Design review of the part built by this model. Coordinates are the model's own, in mm. Give positions to 0.01 mm unless a question says otherwise; leave off trailing zeros. Order: outer loops, then holes, each group sorted by start corner. A loop starts at its lowest first (then second) coordinate and runs counter-clockwise, first axis right, second up. Notation, with made-up numbers: (63.25, -35.5) -> (117.25, -35.5) arc R16 ccw to (117.25, -8.5) -> close; hole circle Ø7 at (-33, 64). An arc over 180 degrees is marked (long way). One line per item, written item: value.
from build123d import *

# Parameters (mm, degrees)
SKETCH1_R          = 16.891
EXTRUDE1_DEPTH     = 7.62
SKETCH2_R          = 8.636
CUT_EXTRUDE4_DEPTH = 26.073415443
SKETCH3_R          = 2.1844
CUT_EXTRUDE6_DEPTH = 7.62
CIRPATTERN1_COUNT  = 6


with BuildPart() as part:
    # Sketch1 → Extrude1 (new body)
    with BuildSketch(Plane(origin=(0, 0, 0), x_dir=(1, 0, 0), z_dir=(0, 1, 0))):
        with Locations(Location((0, 0, 0), (0, 0, 90))):
            Circle(SKETCH1_R)
    extrude(amount=EXTRUDE1_DEPTH)

    # Sketch2 → Cut-Extrude4 (cut, through all)
    with BuildSketch(Plane(origin=(0, 0, 0), x_dir=(1, 0, 0), z_dir=(0, 1, 0))):
        with Locations(Location((0, 0, 0), (0, 0, 90))):
            Circle(SKETCH2_R)
    extrude(amount=CUT_EXTRUDE4_DEPTH, mode=Mode.SUBTRACT)

    # Sketch3 → Cut-Extrude6 (cut)
    with BuildSketch(Plane(origin=(0, 0, 0), x_dir=(1, 0, 0), z_dir=(0, 1, 0))):
        with Locations(Location((0, 13.462, 0), (0, 0, 90))):
            Circle(SKETCH3_R)
    cut_extrude6 = extrude(amount=CUT_EXTRUDE6_DEPTH, mode=Mode.SUBTRACT)

    # CirPattern1: Cut-Extrude6 ×6 about axis
    cirpattern1_axis = Axis((0, 0, 0), (0, 1, 0))
    for i in range(1, CIRPATTERN1_COUNT):
        add(cut_extrude6.rotate(cirpattern1_axis, i * 360 / CIRPATTERN1_COUNT), mode=Mode.SUBTRACT)


solid = part.part
Item 1: Add section C-C on z = 0. Give the boundary of the cut face in (x, y), plus the area to 3 significant figures.
Returned:
outline: (-16.89, 0) -> (-8.64, 0) -> (-8.64, 7.62) -> (-16.89, 7.62) -> close; (8.64, 0) -> (16.89, 0) -> (16.89, 7.62) -> (8.64, 7.62) -> close
area: 126 mm²
Item 2: Add section D-D on x = -5.5. Give the boundary of the cut face in (y, z), plus the area to 3 significant figures.
Returned:
outline: (0, -15.97) -> (7.62, -15.97) -> (7.62, -6.66) -> (0, -6.66) -> close; (0, 6.66) -> (7.62, 6.66) -> (7.62, 15.97) -> (0, 15.97) -> close
area: 142 mm²
Item 3: Add section A-A on z = -7. Give the boundary of the cut face in (x, y), plus the area to 3 significant figures.
Returned:
outline: (-15.37, 0) -> (-13.83, 0) -> (-13.83, 7.62) -> (-15.37, 7.62) -> close; (-9.49, 0) -> (-5.06, 0) -> (-5.06, 7.62) -> (-9.49, 7.62) -> close; (5.06, 0) -> (9.49, 0) -> (9.49, 7.62) -> (5.06, 7.62) -> close; (13.83, 0) -> (15.37, 0) -> (15.37, 7.62) -> (13.83, 7.62) -> close
area: 91.1 mm²
Item 4: Add section B-B on x = 0. Give the boundary of the cut face in (y, z), plus the area to 3 significant figures.
Returned:
outline: (0, -16.89) -> (7.62, -16.89) -> (7.62, -15.65) -> (0, -15.65) -> close; (0, -11.28) -> (7.62, -11.28) -> (7.62, -8.64) -> (0, -8.64) -> close; (0, 8.64) -> (7.62, 8.64) -> (7.62, 11.28) -> (0, 11.28) -> close; (0, 15.65) -> (7.62, 15.65) -> (7.62, 16.89) -> (0, 16.89) -> close
area: 59.2 mm²
Item 5: Draft analysis for pull direction X (two halves, no side actions). For faces 1 (the cylindrical face through (0.84, 3.76, -15.48)), 2 (the cylindrical face through (-5.074, 3.757, -16.111)), 3 (the cylindrical face through (9.72, 3.76, -5.72)), 4 (the flat face through (-8, 0, 4)), state which applies: pulls with the +X half, pulls with the -X half, needs draft (parallel to the pull), parting line crosses it, or undercut.
Returned:
face 1: undercut
face 2: parting line crosses it
face 3: undercut
face 4: needs draft
Item 6: To check wall thickness, follow line 1 along Z through (x, y) = (-13, 4.75); line 2 along Z through (x, y) = (1, 5.5); line 3 along Z through (x, y) = (12.5, 4.5). State the ranges of each line that lie inside material, in increasing order. Write a range as from..to.
Returned:
line 1: -10.78..-8.45, -5.01..5.01, 8.45..10.78
line 2: -16.86..-15.4, -11.52..-8.58, 8.58..11.52, 15.4..16.86
line 3: -11.36..-8.75, -4.72..4.72, 8.75..11.36
Item 7: Clearance check with flat-ended pins moving along their axes: P1, Ø3, axis at x = -4, y = 3, coming from the +Z side; P2, Ø2, axis at y = 1.5, z = -12.5, coming from the -X side; P3, Ø3, axis at y = 5, z = 2, coming from the +X side. State where each tip first meets the part, or that it passes through.
Returned:
P1: z = 16.7
P2: x = -12.37
P3: x = 16.88
